Check sheet for the modelled part. Datum: model origin and axes. Units: mm. Round coordinates to 2 decimals unless told otherwise and drop trailing zeros. Loops run counter-clockwise (first coordinate to the right, second up) from the corner with the lowest first, then second, coordinate; pieces in that order, holes last. Notation, with made-up numbers: (31, 24) - (58, 24) arc R21 cw to (58, 38) - close; hole circle Ø1 at (5.25, -13). An arc over 180 degrees is marked (long way). Put each result on its own line as item: value. Start each with the question number.
```python
from build123d import *

# Parameters (mm, degrees)
SKETCH1_W                                         = 241.3
SKETCH1_H                                         = 22
BASE_FLANGE_DEPTH                                 = 2.5
EDGE_FLANGE_MOUNING_STRIP_W                       = 11.4732
EDGE_FLANGE_MOUNING_STRIP_H                       = 2.5
EDGE_FLANGE_MOUNING_STRIP_CUT_DEPTH               = 219.8
EDGE_FLANGE_MOUNING_RELIEF_W                      = 12.7232
EDGE_FLANGE_MOUNING_RELIEF_H                      = 1.25
EDGE_FLANGE_MOUNING_RELIEF_CUT_DEPTH              = 2.5
EDGE_FLANGE_MOUNING_DEPTH                         = 219.8
CUT_EXTRUDE_MOUNTING_DEPTH                        = 2.5
CSK_FOR_3_FLAT_HEAD_MACHINE_SCREW_100_D           = 2.794
CSK_FOR_3_FLAT_HEAD_MACHINE_SCREW_100_CSINK_D     = 5.0546
CSK_FOR_3_FLAT_HEAD_MACHINE_SCREW_100_CSINK_ANGLE = 100


# Sheet-metal steps are written as plain solids
with BuildPart() as part:
    # Sketch1 → Base-Flange (new body)
    with BuildSketch(Plane.XY):
        with Locations((-120.65, 11)):
            Rectangle(SKETCH1_W, SKETCH1_H)
    extrude(amount=-BASE_FLANGE_DEPTH)

    # Edge-Flange-Mouning strip (across the edge) → Edge-Flange-Mouning strip cut (cut)
    with BuildSketch(Plane(origin=(-219.8, 22, -2.5), x_dir=(0, -1, 0), z_dir=(1, 0, 0))):
        with Locations((-2.5, -1.25)):
            Rectangle(EDGE_FLANGE_MOUNING_STRIP_W, EDGE_FLANGE_MOUNING_STRIP_H)
    extrude(amount=EDGE_FLANGE_MOUNING_STRIP_CUT_DEPTH, mode=Mode.SUBTRACT)

    # Edge-Flange-Mouning relief (on the sheet) → Edge-Flange-Mouning relief cut (cut)
    with BuildSketch(Plane(origin=(-219.8, 18.7634, -2.5), x_dir=(0, -1, 0), z_dir=(0, 0, -1))):
        with Locations((-5.1116, 0.625)):
            Rectangle(EDGE_FLANGE_MOUNING_RELIEF_W, EDGE_FLANGE_MOUNING_RELIEF_H)
    extrude(amount=-EDGE_FLANGE_MOUNING_RELIEF_CUT_DEPTH, mode=Mode.SUBTRACT)

    # Edge-Flange-Mouning section (across the edge) → Edge-Flange-Mouning (add)
    with BuildSketch(Plane(origin=(-219.8, 22, -2.5), x_dir=(0, -1, 0), z_dir=(1, 0, 0))):
        with BuildLine():
            Line((0, 0.7366), (0, 7.5))
            Line((0, 7.5), (2.5, 7.5))
            Line((2.5, 7.5), (2.5, 0.7366))
            ThreePointArc((2.5, 0.7366), (2.715745145, 0.215745145), (3.2366, 0))
            Line((3.2366, 0), (3.2366, -2.5))
            ThreePointArc((3.2366, -2.5), (0.947978192, -1.552021808), (0, 0.7366))
        make_face()
    extrude(amount=EDGE_FLANGE_MOUNING_DEPTH)

    # Sketch13 → Cut-Extrude-Mounting (cut)
    with BuildSketch(Plane.XY):
        with BuildLine():
            Line((-229.5, 12.9), (-235.5, 12.9))
            ThreePointArc((-235.5, 12.9), (-238.5, 15.9), (-235.5, 18.9))
            Line((-235.5, 18.9), (-229.5, 18.9))
            ThreePointArc((-229.5, 18.9), (-226.5, 15.9), (-229.5, 12.9))
        make_face()
    extrude(amount=-CUT_EXTRUDE_MOUNTING_DEPTH, mode=Mode.SUBTRACT)

    # CSK for #3 Flat Head Machine Screw (100)1 (through all)
    with Locations(Plane(origin=(0, 22, 0), x_dir=(1, 0, 0), z_dir=(0, 1, 0))):
        with Locations((-212.8, 7)):
            CounterSinkHole(CSK_FOR_3_FLAT_HEAD_MACHINE_SCREW_100_D / 2, CSK_FOR_3_FLAT_HEAD_MACHINE_SCREW_100_CSINK_D / 2, counter_sink_angle=CSK_FOR_3_FLAT_HEAD_MACHINE_SCREW_100_CSINK_ANGLE)

    # Mirror-Vertical: part across plane


with BuildPart() as part_1:
    add(part.part)
    add(part.part.mirror(Plane(origin=(0, 0, -2.5), x_dir=(0, 0, 1), z_dir=(1, 0, 0))))

    # Mirror-Horizontal: part across face


with BuildPart() as part_2:
    add(part_1.part)
    add(part_1.part.mirror(Plane(origin=(0, 0, -1.25), x_dir=(0, 0, 1), z_dir=(0, -1, 0))))


solid = part_2.part
```
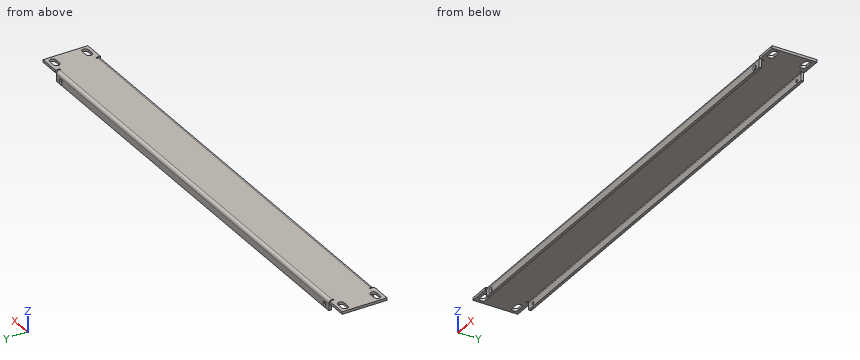
Q1. Cross-section at B-B on y = 9. Enter the section's corners in (x, z), and give its area (3 significant figures).
Q2. Cross-section at A-A on x = -16. Enter the section's corners in (y, z).
Q3. Depth check by flat-ended pin: pin 1 Ø1 at (x, z) = (220.5, -1.5) entering from +Y; pin 2 Ø0.6 at (x, z) = (220.5, -0.5) entering from -Y; pin 3 Ø1 at (x, y) = (-77, -6) entering from -Z; pin 4 Ø2.5 at (x, z) = (-212.8, -7) entering from -Y. Enter the tip coordinate at first touch or a pass-through.
Q4. Material ranges on line 1 (X direction, y = -20.65, z = -7); line 2 (Y direction, x = -147.5, z = -5); line 3 (X direction, y = 20.5, z = -5.5), recorded low to high. Write a range as from..to.
Answer list:
1. outline: (-241.3, -2.5) - (241.3, -2.5) - (241.3, 0) - (-241.3, 0) - close
1. area: 1,210 mm2
2. outline: (-22, -10) - (-19.5, -10) - (-19.5, -3.24) arc R0.74 cw to (-18.76, -2.5) - (18.76, -2.5) arc R0.74 cw to (19.5, -3.24) - (19.5, -10) - (22, -10) - (22, -3.24) arc R3.24 ccw to (18.76, 0) - (-18.76, 0) arc R3.24 ccw to (-22, -3.24) - close
3. pin 1: stops at y = 17.51
3. pin 2: stops at y = -17.51
3. pin 3: stops at z = -2.5
3. pin 4: passes through
4. line 1: x = -219.8..-214.2, -211.4..211.4, 214.2..219.8
4. line 2: y = -22..-19.5, 19.5..22
4. line 3: x = -219.8..219.8
